from build123d import *

# Parameters (mm, degrees)
SKETCH1_R                = 12.7
BOSS_EXTRUDE1_DEPTH      = 4.7752
SKETCH2_R                = 7.1501
BOSS_EXTRUDE2_DEPTH      = 24.13
SKETCH3_R                = 1.8288
BOSS_EXTRUDE3_DEPTH      = 2.54
BOSS_EXTRUDE3_DEPTH_BACK = 17.78


with BuildPart() as part:
    # Sketch1 → Boss-Extrude1 (new body)
    with BuildSketch(Plane.XY):
        Circle(SKETCH1_R)
    extrude(amount=BOSS_EXTRUDE1_DEPTH)

    # Sketch2 → Boss-Extrude2 (add)
    with BuildSketch(Plane(origin=(0, 0, 0), x_dir=(-1, 0, 0), z_dir=(0, 0, -1))):
        Circle(SKETCH2_R)
    extrude(amount=BOSS_EXTRUDE2_DEPTH)

    # Sketch3 → Boss-Extrude3 (add, two sides)
    with BuildSketch(Plane.XY.offset(4.7752)) as boss_extrude3_sk:
        with Locations((0, 9.525)):
            Circle(SKETCH3_R)
        with Locations((8.248891971, 4.7625)):
            Circle(SKETCH3_R)
        with Locations((8.248891971, -4.7625)):
            Circle(SKETCH3_R)
        with Locations((0, -9.525)):
            Circle(SKETCH3_R)
        with Locations((-8.248891971, -4.7625)):
            Circle(SKETCH3_R)
        with Locations((-8.248891971, 4.7625)):
            Circle(SKETCH3_R)
    extrude(amount=BOSS_EXTRUDE3_DEPTH)
    extrude(boss_extrude3_sk.sketch, amount=-BOSS_EXTRUDE3_DEPTH_BACK)


solid = part.part
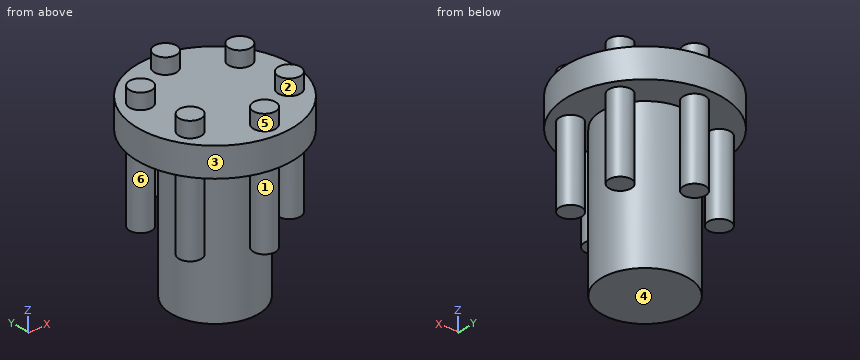
Input: part model. Units: mm. Frame: model coordinates. Face numbers are marked on the shaded views. A direction names the side the tool comes from. Give positions to 0.01 mm unless a question says otherwise; leave off trailing zeros. Order: outer loops, then holes, each group sorted by start corner. A loop starts at its lowest first (then second) coordinate and runs counter-clockwise, first axis right, second up.
Q1. Set-up query: the marked faces 1, 2 and 3. Return all of +Z, -Z, +X, -X, +Y, -Y with unobstructed straight access to the full face (end or side cutting, diameter ignored); none if empty.
Checked values:
face 1: -Z
face 2: +Z
face 3: +Z, -Z
Q2. Section A-A on y = 0. Output: boundary loops of the cut face in (x, z), and give its area (3 significant figures).
Checked values:
outline: (-12.7, 0) - (-7.15, 0) - (-7.15, -24.13) - (7.15, -24.13) - (7.15, 0) - (12.7, 0) - (12.7, 4.78) - (-12.7, 4.78) - close
area: 466 mm2
Q3. Draft query along X for the marked faces 4, 5 and 6. Return one class per face: +X half, -X half, draft (parallel to the pull), parting line (faces both ways), or undercut.
Checked values:
face 4: draft
face 5: parting line
face 6: undercut
Q4. Ray query, probe 1 along X at (y, z) = (-4.25, -4); probe 2 along X at (y, z) = (5.25, -2.5); probe 3 along Y at (x, z) = (-0.25, -6.5). Return the intervals inside material, ascending.
Checked values:
probe 1: x = -10 to -6.49, -5.75 to 5.75, 6.49 to 10
probe 2: x = -10.01 to -6.49, -4.85 to 4.85, 6.49 to 10.01
probe 3: y = -11.34 to -7.71, -7.15 to 7.15, 7.71 to 11.34
Q5. Contact query for flat-ended pins moving along their axis: pin 1 Ø1.5 at (x, y) = (8.5, 10) entering from -Z; pin 2 Ø4 at (x, y) = (9, 5.5) entering from -Z; pin 3 Ø6 at (x, z) = (-7.5, -2) entering from -Y. Output: stop coordinate, or through.
Checked values:
pin 1: stops at z = 0
pin 2: stops at z = -13
pin 3: stops at y = -11.56
Q6. Section C-C on x = 0. Output: boundary loops of the cut face in (y, z), and give its area (3 significant figures).
Checked values:
outline: (-12.7, 0) - (-11.35, 0) - (-11.35, -13) - (-7.7, -13) - (-7.7, 0) - (-7.15, 0) - (-7.15, -24.13) - (7.15, -24.13) - (7.15, 0) - (7.7, 0) - (7.7, -13) - (11.35, -13) - (11.35, 0) - (12.7, 0) - (12.7, 4.78) - (11.35, 4.78) - (11.35, 7.32) - (7.7, 7.32) - (7.7, 4.78) - (-7.7, 4.78) - (-7.7, 7.32) - (-11.35, 7.32) - (-11.35, 4.78) - (-12.7, 4.78) - close
area: 580 mm2
Q7. Section B-B on z = -8. Output: boundary loops of the cut face in (x, y) (1 decimal).
Checked values:
outline: circle Ø3.7 at (-8.2, -4.8); circle Ø3.7 at (-8.2, 4.8); circle Ø14.3 at (0, 0); circle Ø3.7 at (0, -9.5); circle Ø3.7 at (0, 9.5); circle Ø3.7 at (8.2, -4.8); circle Ø3.7 at (8.2, 4.8)
Q8. Section D-D on z = -15. Output: boundary loops of the cut face in (x, y), and give its area (3 significant figures).
Checked values:
outline: circle Ø14.3 at (0, 0)
area: 161 mm2
